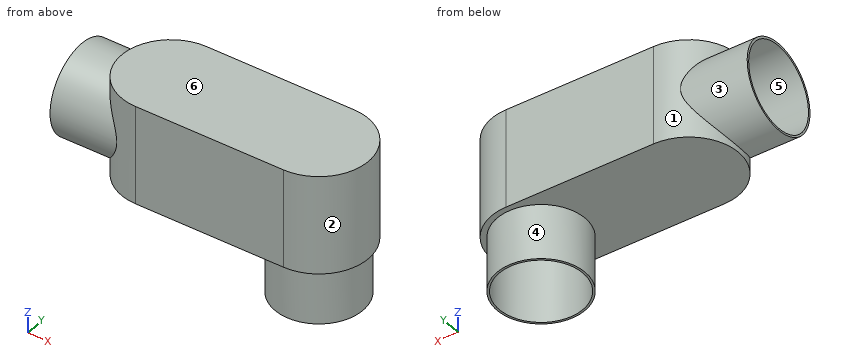
```python
from build123d import *

# Parameters (mm, degrees)
SALIENTE_EXTRUIR1_DEPTH      = 45
SALIENTE_EXTRUIR2_DEPTH      = 25
SALIENTE_EXTRUIR2_DEPTH_BACK = 45
CROQUIS2_R                   = 20
CROQUIS4_R                   = 19.05
CORTAR_EXTRUIR3_DEPTH        = 69
SALIENTE_EXTRUIR3_DEPTH      = 29.495391503
SALIENTE_EXTRUIR3_DEPTH_BACK = 84
CROQUIS5_R                   = 20
CROQUIS8_R                   = 19.05
CORTAR_EXTRUIR6_DEPTH        = 114


with BuildPart() as part:
    # Croquis1 → Saliente-Extruir1 (new body)
    with BuildSketch(Plane.XY):
        with BuildLine():
            Line((-43.5404787, 22.5), (23.3595213, 22.5))
            ThreePointArc((23.3595213, 22.5), (45.8595213, 0), (23.3595213, -22.5))
            Line((23.3595213, -22.5), (-43.5404787, -22.5))
            ThreePointArc((-43.5404787, -22.5), (-66.0404787, 0), (-43.5404787, 22.5))
        make_face()
    extrude(amount=SALIENTE_EXTRUIR1_DEPTH)

    # Croquis2 → Saliente-Extruir2 (add, two sides: drawn at the far end of the back side and taken through both)
    with BuildSketch(Plane(origin=(0, 0, 0), x_dir=(-1, 0, 0), z_dir=(0, 0, -1)).offset(-SALIENTE_EXTRUIR2_DEPTH_BACK)):
        with Locations((-23.3595213, 0)):
            Circle(CROQUIS2_R)
    extrude(amount=SALIENTE_EXTRUIR2_DEPTH + SALIENTE_EXTRUIR2_DEPTH_BACK)

    # Croquis4 → Cortar-Extruir3 (cut)
    with BuildSketch(Plane(origin=(0, 0, -25), x_dir=(-1, 0, 0), z_dir=(0, 0, -1))):
        with Locations((-23.3595213, 0)):
            Circle(CROQUIS4_R)
    extrude(amount=-CORTAR_EXTRUIR3_DEPTH, mode=Mode.SUBTRACT)

    # Croquis5 → Saliente-Extruir3 (add, two sides: drawn at the far end of the back side and taken through both)
    with BuildSketch(Plane(origin=(0, 0, 0), x_dir=(0, 0, -1), z_dir=(1, 0, 0)).offset(-SALIENTE_EXTRUIR3_DEPTH_BACK)):
        with Locations(Location((-22.5, 0, 0), (0, 0, 180))):
            Circle(CROQUIS5_R)
    extrude(amount=SALIENTE_EXTRUIR3_DEPTH + SALIENTE_EXTRUIR3_DEPTH_BACK)

    # Croquis8 → Cortar-Extruir6 (cut)
    with BuildSketch(Plane.ZY.offset(84)):
        with Locations((22.4205324, 0)):
            Circle(CROQUIS8_R)
    extrude(amount=-CORTAR_EXTRUIR6_DEPTH, mode=Mode.SUBTRACT)


solid = part.part
```
Here's how the part is built. I have some questions about the finished solid (model axes, mm). Face numbers are marked on the shaded views. A direction names the side the tool comes from. Give positions to 0.01 mm unless a question says otherwise; leave off trailing zeros. Loops run counter-clockwise (first coordinate to the right, second up) from the corner with the lowest first, then second, coordinate; pieces in that order, holes last. Notation, with made-up numbers: M 59,-20.5 L 110,-20.5 A20 cw 110,-5.5 Z; hole C 66,52.5 d9. An arc over 180 degrees is marked long. Return JSON: item names as keys, results as strings.
Item 1: Imagine slicing it at D-D on z = 22.5. List the corners of the cut face in (x, y) for me, then the cut area to 3 significant figures.
A:
{"outline": "M -84,-20 L -53.85,-20 A22.5 ccw -43.54,-22.5 L 23.36,-22.5 A22.5 ccw 23.36,22.5 L -43.54,22.5 A22.5 ccw -53.85,20 L -84,20 L -84,19.05 L 30,19.05 L 30,17.86 A19.05 cw 30,-17.86 L 30,-19.05 L -84,-19.05 Z", "area": "793 mm^2"}
Item 2: Imagine slicing it at B-B on x = -24. List the corners of the cut face in (y, z) for me, then the cut area to 3 significant figures.
A:
{"outline": "M -22.5,0 L 22.5,0 L 22.5,45 L -22.5,45 Z; hole C 0,22.42 d38.1", "area": "885 mm^2"}
Item 3: On a 3-axis mill with a long thin cutter (end or side, diameter ignored), from which of +Z, -Z, +X, -X, +Y, -Y can I reach the whole of each face in a straight line? I mean the marked faces 1 and 2. Say none if no direction works.
A:
{"face 1": "-X", "face 2": "+Z, -Z, +X"}
Item 4: Please list where these lines run through material, in increasing order: line 1 (Z direction, x = -23, y = 0); line 2 (X direction, y = 11, z = -16); line 3 (Z direction, x = 7, y = -6.5).
A:
{"line 1": "z = 0 to 3.37, 41.47 to 45", "line 2": "x = 6.66 to 7.81, 38.91 to 40.06", "line 3": "z = 3.59 to 4.51, 40.33 to 41.41, 44 to 45"}
Item 5: Imagine slicing it at C-C on x = 19. List the corners of the cut face in (y, z) for me, then the cut area to 3 significant figures.
A:
{"outline": "M -22.5,0 L -19.52,0 L -19.52,-25 L -18.54,-25 L -18.54,15.01 A20 ccw 18.54,15.01 L 18.54,-25 L 19.52,-25 L 19.52,0 L 22.5,0 L 22.5,45 L -22.5,45 Z; hole C 0,22.42 d38.1; hole M -18.54,29.99 A20 cw 18.54,29.99 L 18.54,44 L -18.54,44 Z", "area": "529 mm^2"}
Item 6: I'm going to push flat-ended pins straight in: pin 1 Ø11 at (y, z) = (-3, 32.5) entering from +X; pin 2 Ø6 at (y, z) = (7, 3.5) entering from +X; pin 3 Ø10 at (x, y) = (-59, -15.5) entering from -Z. Where does each tip first touch, or does it pass through?
A:
{"pin 1": "stops at x = 45.86", "pin 2": "stops at x = 45.5", "pin 3": "stops at z = 0"}
Item 7: Imagine slicing it at A-A on y = 0. List the corners of the cut face in (x, z) for me, then the cut area to 3 significant figures.
A:
{"outline": "M -84,2.5 L -66.04,2.5 L -66.04,0 L 3.36,0 L 3.36,-25 L 4.31,-25 L 4.31,2.5 L 29.5,2.5 L 29.5,3.37 L -84,3.37 Z; M -84,41.47 L 29.5,41.47 L 29.5,42.5 L 4.31,42.5 L 4.31,44 L 42.41,44 L 42.41,-25 L 43.36,-25 L 43.36,0 L 45.86,0 L 45.86,45 L -66.04,45 L -66.04,42.5 L -84,42.5 Z", "area": "808 mm^2"}
Item 8: Thinking about a two-plate mould opening in Z: for the marked faces 3, 4, 5 and 6, which applies, released by +Z, released by -Z, zero draft, split by the parting line, or undercut?
A:
{"face 3": "split by the parting line", "face 4": "zero draft", "face 5": "undercut", "face 6": "released by +Z"}
